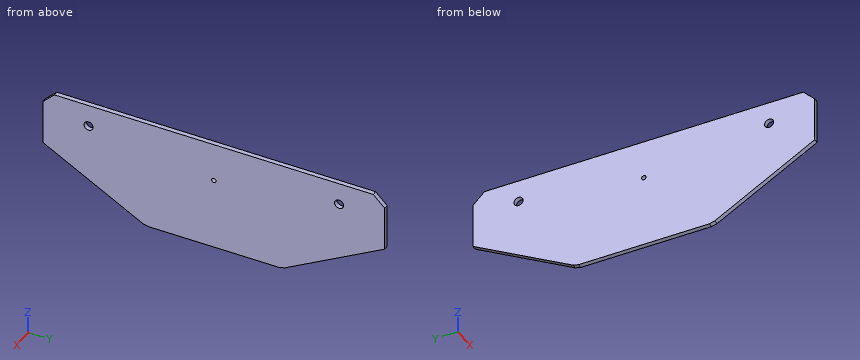
```python
from build123d import *

# Parameters (mm, degrees)
F1_DEPTH    = 2
F3_D        = 8
F5_T1_DEPTH = 55.4336597593
F5_T3_DEPTH = 18.9008056118
F6_D        = 4


# Not quite as in the source:
# - a fillet or chamfer that OpenCascade refuses, or shapes differently, is made with other operations: its cross-section is extruded or revolved along the edge and cut away or added
# - a feature of the source that left no trace in its solid (it failed there, or was rolled back) is left out


with BuildPart() as f1:
    # F0 (on Right) → F1 (new body, symmetric)
    with BuildSketch(Plane.YZ):
        Polygon((150, 100), (-150, 100), (-150, 50), (-60, 0), (60, 0), (150, 50), align=None)
    extrude(amount=F1_DEPTH, both=True)

    # F3 (through all)
    with Locations(Plane.YZ.offset(2)):
        with Locations((-110, 80), (110, 80)):
            Hole(F3_D / 2)

    # F5: chamfer of 10 on 4 edges, made by hand

    # F5_s2 → F5_t1 (cut)
    with BuildSketch(Plane.YZ.offset(-27.7168298797)):
        Polygon((140, 100), (150, 90), (150, 100), align=None)
        Polygon((-140, 100), (-150, 90), (-150, 100), align=None)
    extrude(amount=F5_T1_DEPTH, mode=Mode.SUBTRACT)

    # F5_s4 → F5_t3 (cut)
    with BuildSketch(Plane.YZ.offset(-9.4504028059)):
        Polygon((-62.2651690298, 1.2584272388), (-57.408739718, 0), (-60, 0), align=None)
        Polygon((62.2651690298, 1.2584272388), (57.408739718, 0), (60, 0), align=None)
    extrude(amount=F5_T3_DEPTH, mode=Mode.SUBTRACT)

    # F6 (through all)
    with Locations(Plane.YZ.offset(2)):
        with Locations((0, 65)):
            Hole(F6_D / 2)


solid = f1.part
```
For this review, take the finished solid that the model builds, in its own axes (mm). Coordinates: 2 decimals unless noted, no trailing zeros. Loops run counter-clockwise (first coordinate to the right, second up) from the corner with the lowest first, then second, coordinate; pieces in that order, holes last. Notation, with made-up numbers: (53.5, 48) - (69.5, 48) arc R16 cw to (69.5, 55) - close; hole circle Ø2 at (39.25, -5). An arc over 180 degrees is marked (long way). Use one line per item in the form item = value. Start each with the question number.
1) For pin 1 (5 mm diameter, centred on y = 110, z = 80, fed in from +X); pin 2 (2 mm diameter, centred on x = -1, y = -108, fed in from -Z), all flat-tipped, find the tip position at first contact; note any pin that passes through.
2) Take a section at B-B (x = -0.9). State the section outline as (y, z) points.
3) Take a section at C-C (y = -110). State the section outline as (x, z) points.
4) To check wall thickness, follow probe 1 along Z at (x, y) = (0.2, 0); probe 2 along Z at (x, y) = (-1.05, 110); probe 3 along Y at (x, z) = (-1.8, 30). State the ranges of each line that lie inside material, in increasing order. Write a range as from..to.
5) Take a section at A-A (z = 80). State the section outline as (x, y) points.
6) Take a section at D-D (z = 45.5). State the section outline as (x, y) points, plus the area to 3 significant figures.
From the geometry:
q1.pin_1 = through
q1.pin_2 = 26.11
q2.outline = (-150, 50) - (-62.27, 1.26) - (-57.41, 0) - (57.41, 0) - (62.27, 1.26) - (150, 50) - (150, 90) - (140, 100) - (-140, 100) - (-150, 90) - close; hole circle Ø8 at (-110, 80); hole circle Ø4 at (0, 65); hole circle Ø8 at (110, 80)
q3.outline = (-2, 27.78) - (2, 27.78) - (2, 76) - (-2, 76) - close; (-2, 84) - (2, 84) - (2, 100) - (-2, 100) - close
q4.probe_1 = 0..63, 67..100
q4.probe_2 = 27.78..76, 84..100
q4.probe_3 = -114..114
q5.outline = (-2, -150) - (2, -150) - (2, -114) - (-2, -114) - close; (-2, -106) - (2, -106) - (2, 106) - (-2, 106) - close; (-2, 114) - (2, 114) - (2, 150) - (-2, 150) - close
q6.outline = (-2, -141.9) - (2, -141.9) - (2, 141.9) - (-2, 141.9) - close
q6.area = 1,140 mm2
